Autodesk Inventor part; units mm, degrees
ref_plane "Start Plane" through (0, 0, 0) normal (0, 0, 1) x (1, 0, 0)
ref_plane "End Plane" through (0, 0, 508) normal (0, 0, 1) x (1, 0, 0)
ref_plane "Work Plane4" through (0, -482.6, 0) normal (0, 0, -1) x (-1, 0, 0)
ref_plane "Start Plane" through (0, 0, 0) normal (0, 0, 1) x (1, 0, 0)
ref_plane "End Plane" through (0, 0, 508) normal (0, 0, 1) x (1, 0, 0)
sketch "Sketch" plane through (0, 0, 0) normal (0, 0, 1) x (1, 0, 0)
  line L0 (-25.4, -12.7) -> (-25.4, 12.7)
  line L1 (-12.7, 25.4) -> (12.7, 25.4)
  line L2 (25.4, 12.7) -> (25.4, -12.7)
  line L3 (12.7, -25.4) -> (-12.7, -25.4)
  arc A0 (-25.4, -12.7) -> (-12.7, -25.4) centre (-12.7, -12.7) ccw
  arc A1 (-12.7, 25.4) -> (-25.4, 12.7) centre (-12.7, 12.7) ccw
  arc A2 (25.4, 12.7) -> (12.7, 25.4) centre (12.7, 12.7) ccw
  arc A3 (12.7, -25.4) -> (25.4, -12.7) centre (12.7, -12.7) ccw
  arc A4 (-12.7, 19.05) -> (-19.05, 12.7) centre (-12.7, 12.7) ccw
  line L4 (-12.7, 19.05) -> (12.7, 19.05)
  arc A5 (19.05, 12.7) -> (12.7, 19.05) centre (12.7, 12.7) ccw
  line L5 (19.05, 12.7) -> (19.05, -12.7)
  arc A6 (12.7, -19.05) -> (19.05, -12.7) centre (12.7, -12.7) ccw
  line L6 (12.7, -19.05) -> (-12.7, -19.05)
  arc A7 (-19.05, -12.7) -> (-12.7, -19.05) centre (-12.7, -12.7) ccw
  line L7 (-19.05, -12.7) -> (-19.05, 12.7)
  line L8 (0, 39.2424) -> (0, -39.2424) construction
  line L9 (-39.2424, 0) -> (39.2424, 0) construction
  dimension "d10" = 50.8
  dimension "d11" = 50.8
  dimension "d12" = 6.35
  dimension "d15" = 25.4
  dimension "d16" = 25.4
  dimension "d17" = 12.7
extrude "Body" add sketch "Sketch" along normal up to surface (508 mm away) from surface at 0
sketch "Sketch3" plane through (0, 0, 0) normal (0, 0, 1) x (1, 0, 0)
  line L0 (0, 0) -> (10, 0)
ref_plane "Work Plane3" through (0, 0, 0) normal (0, -1, 0) x (1, 0, 0)
ref_plane "Work Plane4" through (0, -482.6, 0) normal (0, 0, -1) x (-1, 0, 0)
split "Split1" plane through (0, -482.6, 0) removes the side toward (0, 0, -1)
ref_plane "Work Plane5" through (0, -482.6, 508) normal (0, 0, 1) x (1, 0, 0)
split "Split2" plane through (0, -482.6, 508) removes the side toward (0, 0, 1)
ref_plane "Work Plane6" through (25.4, 0, 0) normal (0, 0, -1) x (-1, 0, 0)
split "Split3" plane through (25.4, 0, 0) removes the side toward (0, 0, -1)
ref_plane "Work Plane7" through (25.4, 0, 508) normal (0, 0, 1) x (1, 0, 0)
split "Split4" plane through (25.4, 0, 508) removes the side toward (0, 0, 1)
sketch "Sketch4" plane through (0, 0, 0) normal (0, -1, 0) x (1, 0, 0)
  line L0 (-2, 0) -> (12, 0)
  line L1 (-2, 508) -> (12, 508)
  dimension "d19" = 508
equation "\"d10\" = G_H"
equation "\"d11\" = G_W"
equation "\"d12\" = G_T"
equation "\"d15\" = 0.5 * d10"
equation "\"d16\" = 0.5 * d11"
equation "\"d17\" = G_IR"
equation "\"d3\" = G_L"
equation "\"G_W\" = 50.8"
equation "\"G_H\" = 50.8"
equation "\"G_T\" = 6.35"
equation "\"G_IR\" = 12.7"
equation "\"G_L\" = d19"
equation "\"G_OFFSET_START\" = 0"
equation "\"G_OFFSET_END\" = 0"
equation "\"d14\" = G_OFFSET_END + B_L"
equation "\"B_L\" = 508"
properties part number "AISC - 2 x 2 x 1/4 - 20" material "Steel, Mild"
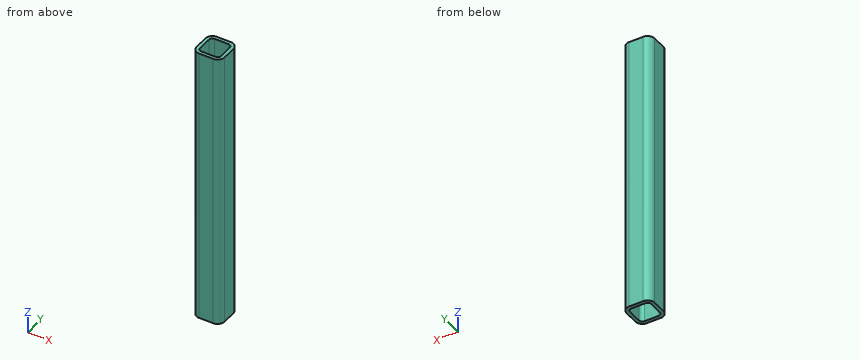
Geometry: final body of the model. Coordinates: model frame, mm. Round coordinates to 2 decimals unless told otherwise and drop trailing zeros. Loops run counter-clockwise (first coordinate to the right, second up) from the corner with the lowest first, then second, coordinate; pieces in that order, holes last. Notation, with made-up numbers: (47, -23.75) - (57, -23.75) arc R16 cw to (57, -8.75) - close; hole circle Ø9 at (70, 25.5). An arc over 180 degrees is marked (long way). Write each question's results on one line, items separated by ' | '. Start each with the question number.
1) Cut plane A-A on y = -7. Return loops of the section in (x, z), then the cut area to 3 significant figures.
2) First-contact query: P1, Ø3, axis at y = 20, z = 80.5, coming from the +X side; P2, Ø8, axis at y = -17, z = 130.5, coming from the -X side. Flat tips, straight axial feed; report the tip coordinate or a pass-through.
3) Cut plane C-C on z = 299.5. Return loops of the section in (x, y), then the cut area to 3 significant figures.
4) Line query: probe 1 along X at (y, z) = (-13.5, 151.5); probe 2 along Y at (x, z) = (11, 163); probe 3 along X at (y, z) = (14.5, 22). Output: solid intervals per line, ascending. Write a range as [from, to].
Verdict:
1) outline: (-25.4, 0) - (-19.05, 0) - (-19.05, 508) - (-25.4, 508) - close; (19.05, 0) - (25.4, 0) - (25.4, 508) - (19.05, 508) - close | area: 6,450 mm2
2) P1: stops at x = 24 | P2: stops at x = -25.4
3) outline: (-25.4, -12.7) arc R12.7 ccw to (-12.7, -25.4) - (12.7, -25.4) arc R12.7 ccw to (25.4, -12.7) - (25.4, 12.7) arc R12.7 ccw to (12.7, 25.4) - (-12.7, 25.4) arc R12.7 ccw to (-25.4, 12.7) - close; hole (-19.05, -12.7) arc R6.35 ccw to (-12.7, -19.05) - (12.7, -19.05) arc R6.35 ccw to (19.05, -12.7) - (19.05, 12.7) arc R6.35 ccw to (12.7, 19.05) - (-12.7, 19.05) arc R6.35 ccw to (-19.05, 12.7) - close | area: 1,030 mm2
4) probe 1: x = [-25.37, -19], [19, 25.37] | probe 2: y = [-25.4, -19.05], [19.05, 25.4] | probe 3: x = [-25.27, -18.79], [18.79, 25.27]
